```python
from build123d import *

# Parameters (mm, degrees)
SKETCH1_W                                      = 80
SKETCH1_H                                      = 25.3
BOSS_EXTRUDE1_DEPTH                            = 3.2
CSK_FOR_M5_FLAT_HEAD_MACHINE_SCREW1_AT_2_COUNT = 2
CSK_FOR_M5_FLAT_HEAD_MACHINE_SCREW1_AT_2_PITCH = 44


with BuildPart() as part:
    # Sketch1 → Boss-Extrude1 (new body)
    with BuildSketch(Plane(origin=(0, 0, 0), x_dir=(1, 0, 0), z_dir=(0, 1, 0))):
        with Locations((40, -12.65)):
            Rectangle(SKETCH1_W, SKETCH1_H)
    extrude(amount=BOSS_EXTRUDE1_DEPTH)

    # Sketch3 → CSK for M5 Flat Head Machine Screw1 (revolve, cut)
    with BuildSketch(Plane(origin=(62, 0, 12.65), x_dir=(0, 0, -1), z_dir=(1, 0, 0))):
        Polygon((0, 0), (0, 3.2), (2.75, 3.2), (2.75, 2.45), (5.2, 0), align=None)
    csk_for_m5_flat_head_machine_screw1 = revolve(axis=Axis((62, -6.35, 12.65), (0, 1, 0)), mode=Mode.SUBTRACT)

    # CSK for M5 Flat Head Machine Screw1 at 2: CSK for M5 Flat Head Machine Screw1 ×2
    with Locations(*[(-i * CSK_FOR_M5_FLAT_HEAD_MACHINE_SCREW1_AT_2_PITCH, 0, 0) for i in range(1, CSK_FOR_M5_FLAT_HEAD_MACHINE_SCREW1_AT_2_COUNT)]):
        add(csk_for_m5_flat_head_machine_screw1, mode=Mode.SUBTRACT)


solid = part.part
```
Part model, mm, in its own coordinate system. Coordinates: 2 decimals unless noted, no trailing zeros. Loops run counter-clockwise (first coordinate to the right, second up) from the corner with the lowest first, then second, coordinate; pieces in that order, holes last. Notation, with made-up numbers: (-32.75, 69) - (-14.75, 69) arc R34 ccw to (-14.75, 102) - close; hole circle Ø5 at (25.25, 47). An arc over 180 degrees is marked (long way). Write item = value, one per line. Start each with the question number.
Item 1: Cut at A-A, the plane z = 12.65. Give the cut face in (x, y).
Item 2: Wall check: L1, parallel to X at y = 2.8, z = 12.65; L2, parallel to Z at x = 62, y = 2.6; L3, parallel to X at y = 0.6, z = 8.5. Give the ranges that are in metal, low to high. Write a range as from..to.
Item 3: Mould opens along Z. For faces 1 (the flat face through (39, 3.2, 12)), 2 (the flat face through (39, 2, 0)), 3 (the cylindrical face through (59.273, 2.82, 13.008)) say: released by +Z, released by -Z, zero draft, split by the parting line, or undercut.
Item 4: Cut at B-B, the plane x = 62. Give the cut face in (y, z), and give its area (3 significant figures).
Item 5: Cut at C-C, the plane y = 1.25. Give the cut face in (x, z), and give its area (3 significant figures).
The answers:
q1.outline = (0, 0) - (12.8, 0) - (15.25, 2.45) - (15.25, 3.2) - (0, 3.2) - close; (20.75, 2.45) - (23.2, 0) - (56.8, 0) - (59.25, 2.45) - (59.25, 3.2) - (20.75, 3.2) - close; (64.75, 2.45) - (67.2, 0) - (80, 0) - (80, 3.2) - (64.75, 3.2) - close
q2.L1 = 0..15.25, 20.75..59.25, 64.75..80
q2.L2 = 0..9.9, 15.4..25.3
q2.L3 = 0..16.02, 19.98..60.02, 63.98..80
q3.face_1 = zero draft
q3.face_2 = released by -Z
q3.face_3 = undercut
q4.outline = (0, 0) - (3.2, 0) - (3.2, 9.9) - (2.45, 9.9) - (0, 7.45) - close; (0, 17.85) - (2.45, 15.4) - (3.2, 15.4) - (3.2, 25.3) - (0, 25.3) - close
q4.area = 57.4 mm2
q5.outline = (0, 0) - (80, 0) - (80, 25.3) - (0, 25.3) - close; hole circle Ø7.9 at (18, 12.65); hole circle Ø7.9 at (62, 12.65)
q5.area = 1,930 mm2
